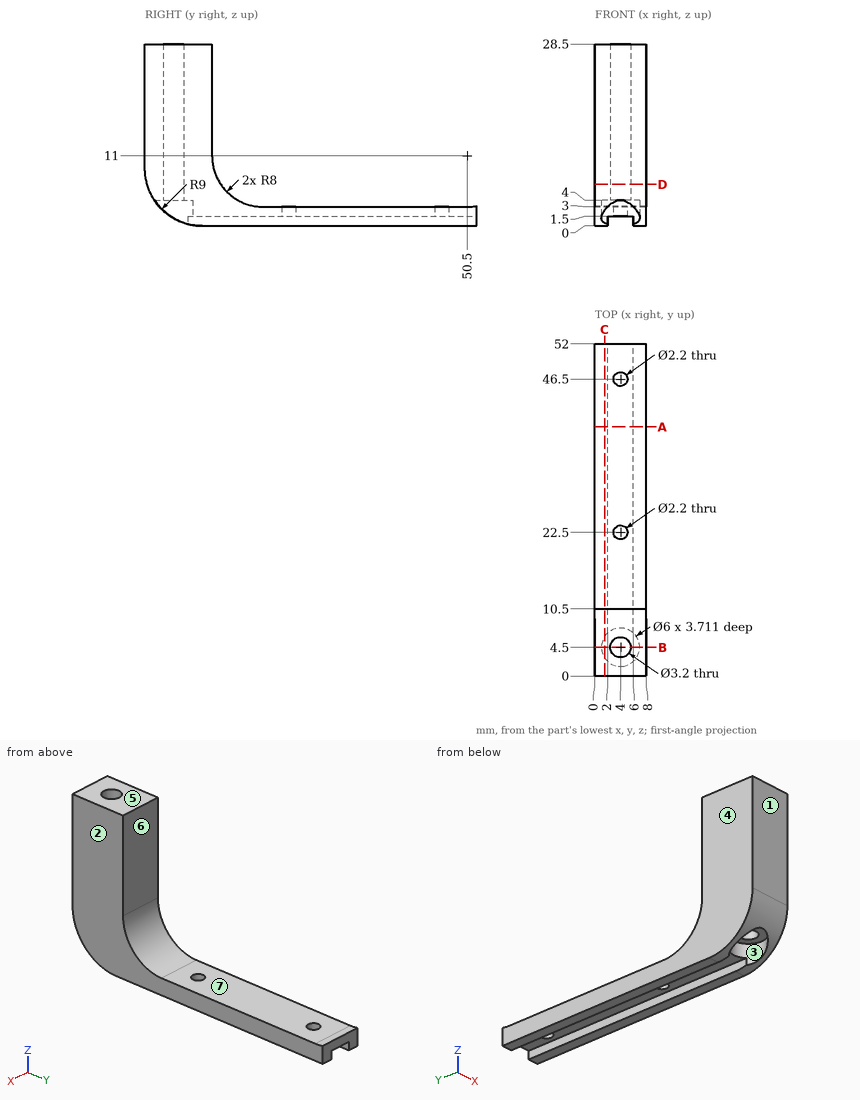
The figure shows three views and two pictorial views of one solid part (mm, origin at its lowest corner). Answer the questions. A direction names the side the tool comes from. Give positions to 0.01 mm unless a question says otherwise; leave off trailing zeros. Order: outer loops, then holes, each group sorted by start corner. A loop starts at its lowest first (then second) coordinate and runs counter-clockwise, first axis right, second up. Notation, with made-up numbers: M 79.5,35.25 L 99.5,35.25 A16 cw 99.5,62.25 Z; hole C 2.25,52 d9. An arc over 180 degrees is marked long. Return JSON: item names as keys, results as strings.
1) Straight lines are drawn through the part: line 1 along Y through (x, z) = (4, 2.6); line 2 along Y through (x, z) = (4, 21.5); line 3 along X through (y, z) = (4.5, 3.15). For each, find the intervals that lie inside material, in ascending order. Write a range as [from, to].
Resolved:
{"line 1": "[7.5, 21.4], [23.6, 45.4], [47.6, 52]", "line 2": "[0, 2.9], [6.1, 10.5]", "line 3": "[0, 1], [7, 8]"}
2) Section B-B, the plane y = 4.5 is taken. Write down the section's boundary in (x, z) (1 decimal).
Resolved:
{"outline": "M 0,1.2 L 1,1.2 L 1,4 L 2.4,4 L 2.4,28.5 L 0,28.5 Z; M 5.6,4 L 7,4 L 7,1.2 L 8,1.2 L 8,28.5 L 5.6,28.5 Z"}
3) Section C-C, the plane x = 1.5 is taken. Write down the section's boundary in (y, z), plus the area to 3 significant figures.
Resolved:
{"outline": "M 0,9 A9 ccw 2.84,2.44 L 2.84,4 L 6.16,4 L 6.16,0.46 A9 ccw 9,0 L 52,0 L 52,3.14 A8 cw 50.5,3 L 18.5,3 A8 cw 10.5,11 L 10.5,28.5 L 0,28.5 Z", "area": "411 mm^2"}
4) For a pull along X with two mould halves and no side action, classify the marked faces 1, 2, 3 and 4 as +X half, -X half, draft (parallel to the pull), parting line (faces both ways), or undercut.
Resolved:
{"face 1": "draft", "face 2": "+X half", "face 3": "undercut", "face 4": "-X half"}
5) Section D-D, the plane z = 6.5 is taken. Write down the section's boundary in (x, y) (1 decimal).
Resolved:
{"outline": "M 0,0.4 L 8,0.4 L 8,11.9 L 0,11.9 Z; hole C 4,4.5 d3.2"}
6) Each of these flat-tipped pins is pushed along its axis until it touches: pin 1 (1 mm diameter, centred on x = 3.5, z = 12.5, fed in from +Y); pin 2 (1 mm diameter, centred on x = 5, y = 28.5, fed in from -Z); pin 3 (3 mm diameter, centred on x = 4.5, y = 41, fed in from +Z). Where does it stop, or does it pass through?
Resolved:
{"pin 1": "y = 10.5", "pin 2": "z = 1.5", "pin 3": "z = 3"}
7) A tool of negligible diameter and unlimited length cuts with its end or side. For the marked faces 5, 6 and 7, from which of +Z, -Z, +X, -X, +Y, -Y can it reach the whole face along a straight path? Write none if from no direction.
Resolved:
{"face 5": "+Z, +X, -X, +Y, -Y", "face 6": "+Z, +X, -X, +Y", "face 7": "+Z, +X, -X"}
8) Section A-A, the plane y = 39 is taken. Write down the section's boundary in (x, z).
Resolved:
{"outline": "M 0,0 L 2,0 L 2,1.5 L 6,1.5 L 6,0 L 8,0 L 8,3 L 0,3 Z"}
